from build123d import *

# Parameters (mm, degrees)
F0_R     = 3.3625011168
F1_DEPTH = 111.76


# Not quite as in the source:
# - ends of sketch curves that miss each other by under 0.0002 mm in the source are joined


with BuildPart() as f1:
    # F0 (on Top) → F1 (new body)
    with BuildSketch(Plane.XY):
        with BuildLine():
            ThreePointArc((3.5659002011, 5.7489795053), (2.3298472421, 4.9230753228), (0.8718233648, 4.6330563417))
            Line((0.8718233648, 4.6330563417), (-2.0428700475, 4.6330563417))
            ThreePointArc((-2.0428700475, 4.6330563417), (-3.5008939248, 4.9230753228), (-4.7369468838, 5.7489795053))
            Line((-4.7369468838, 5.7489795053), (-6.5824285393, 7.5944611609))
            ThreePointArc((-6.5824285393, 7.5944611609), (-6.9953806306, 9.6705115177), (-5.2353901211, 10.846499579))
            Line((-5.2353901211, 10.846499579), (-3.5008939248, 10.846499579))
            Line((-3.5008939248, 10.846499579), (-3.4685428807, 10.846499579))
            ThreePointArc((-3.4685428807, 10.846499579), (-2.7109282724, 11.6201206221), (-3.4685428807, 12.3937416652))
            Line((-3.4685428807, 12.3937416652), (-3.5008939248, 12.3937416652))
            Line((-3.5008939248, 12.3937416652), (-4.1388643307, 12.3937416652))
            ThreePointArc((-4.1388643307, 12.3937416652), (-4.6871272259, 11.8525139305), (-5.2353901211, 12.3937416652))
            Line((-5.2353901211, 12.3937416652), (-8.3730050695, 12.3937416652))
            ThreePointArc((-8.3730050695, 12.3937416652), (-8.9242642054, 11.8424825293), (-9.4755233413, 12.3937416652))
            ThreePointArc((-9.4755233413, 12.3937416652), (-12.1696001777, 11.2778185015), (-13.2855233413, 8.5837416652))
            Line((-13.2855233413, 8.5837416652), (-13.2855233413, 7.4984658996))
            Line((-13.2855233413, 7.4984658996), (-13.2855233413, 4.343608445))
            ThreePointArc((-13.2855233413, 4.343608445), (-12.7296839168, 3.7964165708), (-13.2855233413, 3.2492246965))
            Line((-13.2855233413, 3.2492246965), (-13.2855233413, 2.6091122487))
            ThreePointArc((-13.2855233413, 2.6091122487), (-12.5119022982, 1.8532957784), (-11.7382812551, 2.6091122487))
            Line((-11.7382812551, 2.6091122487), (-11.7382812551, 4.343608445))
            ThreePointArc((-11.7382812551, 4.343608445), (-10.5622931938, 6.1035989545), (-8.486242837, 5.6906468632))
            Line((-8.486242837, 5.6906468632), (-6.6407611815, 3.8451652077))
            ThreePointArc((-6.6407611815, 3.8451652077), (-5.8148569989, 2.6091122487), (-5.5248380178, 1.1510883714))
            Line((-5.5248380178, 1.1510883714), (-5.5248380178, -1.7636050409))
            ThreePointArc((-5.5248380178, -1.7636050409), (-5.8148569989, -3.2216289182), (-6.6407611815, -4.4576818772))
            Line((-6.6407611815, -4.4576818772), (-8.486242837, -6.3031635328))
            ThreePointArc((-8.486242837, -6.3031635328), (-10.5622931938, -6.716115624), (-11.7382812551, -4.9561251146))
            Line((-11.7382812551, -4.9561251146), (-11.7382812551, -3.2216289182))
            ThreePointArc((-11.7382812551, -3.2216289182), (-12.5119022982, -2.4480078751), (-13.2855233413, -3.2216289182))
            Line((-13.2855233413, -3.2216289182), (-13.2855233413, -3.8570189362))
            Line((-13.2855233413, -3.8570189362), (-13.2855233413, -3.8595993241))
            ThreePointArc((-13.2855233413, -3.8595993241), (-12.7442956066, -4.4078622194), (-13.2855233413, -4.9561251146))
            Line((-13.2855233413, -4.9561251146), (-13.2855233413, -8.093740063))
            ThreePointArc((-13.2855233413, -8.093740063), (-12.9963771793, -8.175658031), (-12.7931661592, -8.3970656592))
            ThreePointArc((-12.7931661592, -8.3970656592), (-12.8130701183, -8.9360625991), (-13.2855233413, -9.1962583348))
            ThreePointArc((-13.2855233413, -9.1962583348), (-12.1696001777, -11.8903351711), (-9.4755233413, -13.0062583348))
            ThreePointArc((-9.4755233413, -13.0062583348), (-8.9263401234, -12.4513735034), (-8.3771569056, -13.0062583348))
            Line((-8.3771569056, -13.0062583348), (-5.2353901211, -13.0062583348))
            ThreePointArc((-5.2353901211, -13.0062583348), (-4.6881982469, -12.4504189103), (-4.1410063726, -13.0062583348))
            Line((-4.1410063726, -13.0062583348), (-3.5008939248, -13.0062583348))
            ThreePointArc((-3.5008939248, -13.0062583348), (-2.7450774545, -12.2326372917), (-3.5008939248, -11.4590162486))
            Line((-3.5008939248, -11.4590162486), (-5.2353901211, -11.4590162486))
            ThreePointArc((-5.2353901211, -11.4590162486), (-6.9953806306, -10.2830281872), (-6.5824285393, -8.2069778304))
            ThreePointArc((-6.5824285393, -8.2069778304), (-6.5813491493, -8.2058993046), (-6.5802706255, -8.2048199166))
            Line((-6.5802706255, -8.2048199166), (-4.7369468838, -6.3614961749))
            ThreePointArc((-4.7369468838, -6.3614961749), (-3.5008939248, -5.5355919924), (-2.0428700475, -5.2455730112))
            Line((-2.0428700475, -5.2455730112), (0.8718233648, -5.2455730112))
            ThreePointArc((0.8718233648, -5.2455730112), (2.3298472421, -5.5355919924), (3.5659002011, -6.3614961749))
            Line((3.5659002011, -6.3614961749), (5.4092239428, -8.2048199166))
            ThreePointArc((5.4092239428, -8.2048199166), (5.8221760341, -10.2808702734), (4.0621855247, -11.4568583348))
            Line((4.0621855247, -11.4568583348), (2.3298472421, -11.4568583348))
            ThreePointArc((2.3298472421, -11.4568583348), (1.7126411358, -12.2315583348), (2.3298472421, -13.0062583348))
            Line((2.3298472421, -13.0062583348), (2.9616088274, -13.0062583348))
            ThreePointArc((2.9616088274, -13.0062583348), (3.511897176, -12.460996221), (4.0621855247, -13.0062583348))
            Line((4.0621855247, -13.0062583348), (7.2156104858, -13.0062583348))
            ThreePointArc((7.2156104858, -13.0062583348), (7.7600435722, -12.4618252483), (8.3044766587, -13.0062583348))
            ThreePointArc((8.3044766587, -13.0062583348), (10.998553495, -11.8903351711), (12.1144766587, -9.1962583348))
            ThreePointArc((12.1144766587, -9.1962583348), (11.5750962663, -8.6501583348), (12.1144766587, -8.1040583348))
            Line((12.1144766587, -8.1040583348), (12.1144766587, -4.9539672008))
            ThreePointArc((12.1144766587, -4.9539672008), (11.570959409, -4.4045980675), (12.1144766587, -3.8552289343))
            Line((12.1144766587, -3.8552289343), (12.1144766587, -3.2216289182))
            ThreePointArc((12.1144766587, -3.2216289182), (11.3397766587, -2.5015675684), (10.5650766587, -3.2216289182))
            Line((10.5650766587, -3.2216289182), (10.5650766587, -4.9539672008))
            ThreePointArc((10.5650766587, -4.9539672008), (9.3890885973, -6.7139577102), (7.3130382405, -6.301005619))
            Line((7.3130382405, -6.301005619), (5.4697144988, -4.4576818772))
            ThreePointArc((5.4697144988, -4.4576818772), (4.6438103163, -3.2216289182), (4.3537913351, -1.7636050409))
            Line((4.3537913351, -1.7636050409), (4.3537913351, 1.1510883714))
            ThreePointArc((4.3537913351, 1.1510883714), (4.6438103163, 2.6091122487), (5.4697144988, 3.8451652077))
            Line((5.4697144988, 3.8451652077), (7.3130382405, 5.6884889494))
            ThreePointArc((7.3130382405, 5.6884889494), (9.3890885973, 6.1014410407), (10.5650766587, 4.3414505312))
            Line((10.5650766587, 4.3414505312), (10.5650766587, 2.6091122487))
            ThreePointArc((10.5650766587, 2.6091122487), (11.3397766587, 1.8731471479), (12.1144766587, 2.6091122487))
            Line((12.1144766587, 2.6091122487), (12.1144766587, 3.2492505312))
            ThreePointArc((12.1144766587, 3.2492505312), (11.5683766587, 3.7953505312), (12.1144766587, 4.3414505312))
            Line((12.1144766587, 4.3414505312), (12.1144766587, 7.4889068047))
            ThreePointArc((12.1144766587, 7.4889068047), (11.563421032, 8.0363242349), (12.1144766587, 8.5837416652))
            ThreePointArc((12.1144766587, 8.5837416652), (10.998553495, 11.2778185015), (8.3044766587, 12.3937416652))
            ThreePointArc((8.3044766587, 12.3937416652), (7.7491737928, 11.89736095), (7.1938709268, 12.3937416652))
            Line((7.1938709268, 12.3937416652), (4.0643434385, 12.3937416652))
            ThreePointArc((4.0643434385, 12.3937416652), (3.5181119113, 11.8531747523), (2.9718803841, 12.3937416652))
            Line((2.9718803841, 12.3937416652), (2.3298472421, 12.3937416652))
            Line((2.3298472421, 12.3937416652), (2.2582739116, 12.3937416652))
            ThreePointArc((2.2582739116, 12.3937416652), (1.5196122547, 11.6201206221), (2.2582739116, 10.846499579))
            Line((2.2582739116, 10.846499579), (2.3298472421, 10.846499579))
            Line((2.3298472421, 10.846499579), (4.0643434385, 10.846499579))
            ThreePointArc((4.0643434385, 10.846499579), (5.8243339479, 9.6705115177), (5.4113818566, 7.5944611609))
            Line((5.4113818566, 7.5944611609), (3.5659002011, 5.7489795053))
        make_face()
        with Locations((-0.5855233413, -0.3062583348)):
            Circle(F0_R, mode=Mode.SUBTRACT)
    extrude(amount=F1_DEPTH)


solid = f1.part
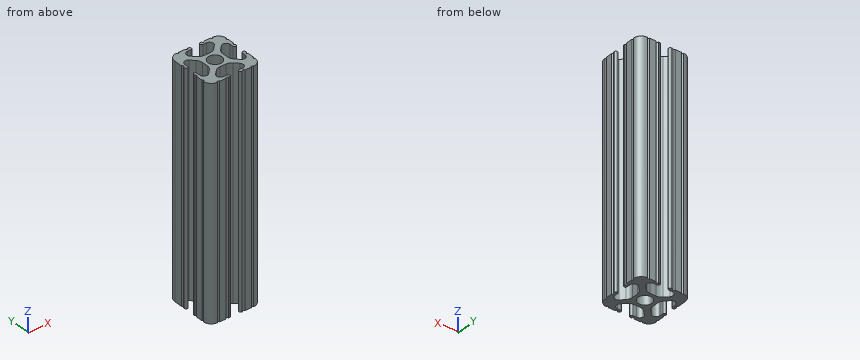
The model under review builds one solid part; all positions refer to its coordinate system, in mm. Round coordinates to 2 decimals unless told otherwise and drop trailing zeros. Loops run counter-clockwise (first coordinate to the right, second up) from the corner with the lowest first, then second, coordinate; pieces in that order, holes last. Notation, with made-up numbers: M -7,54 L 31,54 A15 cw 31,80 Z; hole C 33,-6 d2. An arc over 180 degrees is marked long. Answer as a JSON object with one key per item and string values.
Item 1: We need section A-A, the plane x = -10.5. State the section outline as (y, z) points, and give its area (3 significant figures).
Check sheet entries:
{"outline": "M -12.87,0 L -6.74,0 L -6.74,111.76 L -12.87,111.76 Z; M 6.13,0 L 12.25,0 L 12.25,111.76 L 6.13,111.76 Z", "area": "1,370 mm2"}
Item 2: Clearance check with flat-ended pins moving along their axes: P1, Ø3, axis at x = -1, z = 73, coming from the -Y side; P2, Ø0.9, axis at y = -0.5, z = 54.5, coming from the +X side; P3, Ø2.5, axis at x = 0, z = 33, coming from the +Y side. State where each tip first meets the part, or that it passes through.
Check sheet entries:
{"P1": "y = -5.27", "P2": "x = 4.35", "P3": "y = 4.65"}
Item 3: For line 1 along X through (y, z) = (2, 97); line 2 along Y through (x, z) = (5, 54); line 3 along Y through (x, z) = (5.5, 27), list the stretches that pass through material, from the lowest coordinate up.
Check sheet entries:
{"line 1": "-12.97 to -12.06, -5.62 to -3.03, 1.86 to 4.45, 10.91 to 11.76", "line 2": "-13.01 to -11.21, -7.8 to -3.89, 3.27 to 7.18, 10.6 to 12.39", "line 3": "-13.01 to -10.8, -8.3 to -4.49, 3.88 to 7.69, 10.19 to 12.39"}
